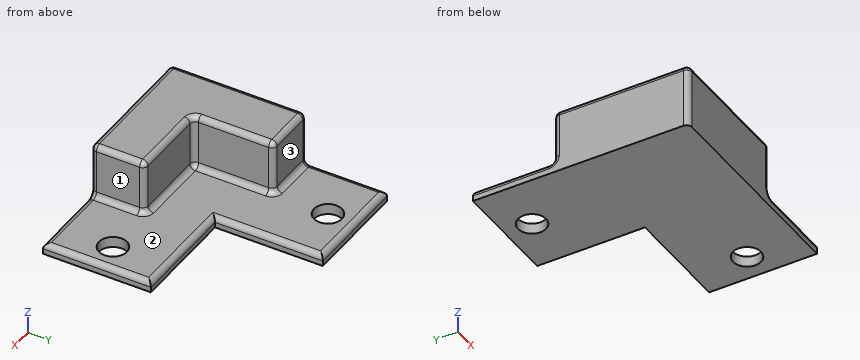
from build123d import *

# Parameters (mm, degrees)
SKETCH1_R           = 2.6
BOSS_EXTRUDE1_DEPTH = 2
BOSS_EXTRUDE2_DEPTH = 10
FILLET1_R           = 1


with BuildPart() as part:
    # Sketch1 → Boss-Extrude1 (new body)
    with BuildSketch(Plane.XY):
        Polygon((0, 20), (0, 0), (20, 0), (20, -20), (-20, -20), (-20, 20), align=None)
        with Locations((-10, 15)):
            Circle(SKETCH1_R, mode=Mode.SUBTRACT)
        with Locations((15, -10)):
            Circle(SKETCH1_R, mode=Mode.SUBTRACT)
    extrude(amount=BOSS_EXTRUDE1_DEPTH)

    # Sketch2 → Boss-Extrude2 (add)
    with BuildSketch(Plane.XY.offset(2)):
        Polygon((-10, 5), (-20, 5), (-20, -20), (5, -20), (5, -10), (-10, -10), align=None)
    extrude(amount=BOSS_EXTRUDE2_DEPTH)

    # Fillet1
    fillet1_edges = [part.edges().sort_by_distance(p)[0] for p in [
        (-20, -20, 6),
        (20, -10, 2),
        (10, 0, 2),
        (0, 10, 2),
        (-10, 20, 2),
        (12.5, -20, 2),
        (-10, -2.5, 2),
        (-10, -10, 7),
        (-15, 5, 2),
        (-10, 5, 7),
        (-20, 5, 7),
        (5, -15, 2),
        (5, -20, 7),
        (-2.5, -10, 2),
        (5, -10, 7),
        (-10, -2.5, 12),
        (-15, 5, 12),
        (-20, -7.5, 12),
        (-7.5, -20, 12),
        (5, -15, 12),
        (-2.5, -10, 12),
        (-20, 12.5, 2),
    ]]
    fillet(fillet1_edges, radius=FILLET1_R)


solid = part.part
Verification items for the finished model (mm, model axes). Face numbers are marked on the shaded views. A direction names the side the tool comes from. Coordinates: 2 decimals unless noted, no trailing zeros. Loops run counter-clockwise (first coordinate to the right, second up) from the corner with the lowest first, then second, coordinate; pieces in that order, holes last. Notation, with made-up numbers: (68.5, 65) -> (96.5, 65) arc R13 cw to (96.5, 72) -> close; hole circle Ø4 at (-10, -7). An arc over 180 degrees is marked (long way). Answer as CSV lines item,"result".
1) Depth check by flat-ended pin: pin 1 (6.5 mm diameter, centred on x = -14, z = 5.5, fed in from +Y); pin 2 (1 mm diameter, centred on x = -8.5, z = 7, fed in from +Y); pin 3 (5 mm diameter, centred on y = -13, z = 5.5, fed in from +X). Enter the tip coordinate at first touch or a pass-through.
Found:
pin 1,"stops at y = 5.34"
pin 2,"stops at y = -10"
pin 3,"stops at x = 5"
2) Cross-section at D-D, the plane x = 7. Record the cut outline in (y, z), then the cut area to 3 significant figures.
Found:
outline,"(-20, 0) -> (0, 0) -> (0, 1) arc R1 ccw to (-1, 2) -> (-19, 2) arc R1 ccw to (-20, 1) -> close"
area,"39.6 mm2"
3) Tool access check on the marked faces 1, 2 and 3. Record the directions out of +Z, -Z, +X, -X, +Y, -Y that give a thin tool (end or side, any length) a straight path to the whole face; none if there is none.
Found:
face 1,"+Z, +X, +Y, -Y"
face 2,"+Z, +X, +Y"
face 3,"+Z, +X, -X, +Y"
4) Cross-section at C-C, the plane z = 6. Record the cut outline in (x, y).
Found:
outline,"(-20, -19) arc R1 ccw to (-19, -20) -> (4, -20) arc R1 ccw to (5, -19) -> (5, -11) arc R1 ccw to (4, -10) -> (-9, -10) arc R1 cw to (-10, -9) -> (-10, 4) arc R1 ccw to (-11, 5) -> (-19, 5) arc R1 ccw to (-20, 4) -> close"
5) Thickness scan on L1, parallel to Y at x = 15, z = 0.9; L2, parallel to Y at x = -10, z = 0.6; L3, parallel to Y at x = -15, z = 9. Record the ranges inside material, lowest first. Write a range as from..to.
Found:
L1,"y = -20..-12.6, -7.4..0"
L2,"y = -20..12.4, 17.6..20"
L3,"y = -20..5"
6) Cross-section at A-A, the plane x = 15. Record the cut outline in (y, z), then the cut area to 3 significant figures.
Found:
outline,"(-20, 0) -> (-12.6, 0) -> (-12.6, 2) -> (-19, 2) arc R1 ccw to (-20, 1) -> close; (-7.4, 0) -> (0, 0) -> (0, 1) arc R1 ccw to (-1, 2) -> (-7.4, 2) -> close"
area,"29.2 mm2"
